The listing builds one solid part. Answer for the finished solid, in the listing's coordinates (mm). Face numbers are marked on the shaded views. A direction names the side the tool comes from. Coordinates: 2 decimals unless noted, no trailing zeros. Order: outer loops, then holes, each group sorted by start corner. A loop starts at its lowest first (then second) coordinate and runs counter-clockwise, first axis right, second up. Notation, with made-up numbers: (52.5, -15.75) -> (68.5, -15.75) arc R12 cw to (68.5, 0.25) -> close; hole circle Ø8 at (-35.75, 27). An arc over 180 degrees is marked (long way). Put each result on its own line as item: value. Start each with the question number.
Autodesk Inventor part; units mm, degrees
ref_plane "YZ Plane" through (0, 0, 0) normal (1, 0, 0) x (0, 1, 0)
ref_plane "XZ Plane" through (0, 0, 0) normal (0, 1, 0) x (-1, 0, 0)
ref_plane "XY Plane" through (0, 0, 0) normal (0, 0, 1) x (1, 0, 0)
sketch "Эскиз1" plane through (0, 0, 0) normal (0, 0, 1) x (1, 0, 0)
  line L0 (-26, 14.5) -> (26, 14.5)
  line L1 (26, 14.5) -> (26, -14.5)
  line L2 (26, -14.5) -> (-26, -14.5)
  line L3 (-26, -14.5) -> (-26, 14.5)
  line L4 (0, -20.3) -> (0, 20.3)
  line L5 (-36.4, 0) -> (36.4, 0)
  point P0 (0, 0)
  dimension "d0" = 29
  dimension "d1" = 52
extrude "Выдавливание1" add sketch "Эскиз1" along normal blind 2
sketch "Эскиз2" plane through (0, 0, 2) normal (0, 0, 1) x (1, 0, 0)
  line L0 (-26, 14.5) -> (-26, -14.5)
  line L1 (26, 14.5) -> (-26, 14.5)
  line L2 (26, -14.5) -> (26, 14.5)
  line L3 (-26, -14.5) -> (26, -14.5)
  line L4 (-26, 14.5) -> (26, 14.5)
  line L5 (26, 14.5) -> (26, -14.5)
  line L6 (26, -14.5) -> (-26, -14.5)
  line L7 (-26, -14.5) -> (-26, 14.5)
  line L8 (-25, 13.5) -> (25, 13.5)
  line L9 (25, 13.5) -> (25, -13.5)
  line L10 (25, -13.5) -> (-25, -13.5)
  line L11 (-25, -13.5) -> (-25, 13.5)
  point P0 (0, 0)
  dimension "d4" = 1
  dimension "d5" = 1
  dimension "d6" = 1
  dimension "d7" = 1
extrude "Выдавливание2" add sketch "Эскиз2" along normal blind 15
sketch "Эскиз3" plane through (0, 0, 17) normal (0, 0, 1) x (1, 0, 0)
  line L0 (-26, 14.5) -> (-26, -14.5)
  line L1 (-26, 14.5) -> (-26, 14.5)
  line L2 (-26, 14.5) -> (-26, -14.5)
  line L3 (-26, -14.5) -> (-26, -14.5)
  line L4 (-28, -12.5) -> (-28, 12.5)
  line L5 (26, 14.5) -> (-26, 14.5)
  line L6 (26, 14.5) -> (26, 14.5)
  line L7 (28, 12.5) -> (28, -12.5)
  line L8 (26, -14.5) -> (26, -14.5)
  line L9 (26, -14.5) -> (26, 14.5)
  arc A0 (-26, 14.5) -> (-28, 12.5) centre (-26, 12.5) ccw
  arc A1 (-28, -12.5) -> (-26, -14.5) centre (-26, -12.5) ccw
  arc A2 (26, -14.5) -> (28, -12.5) centre (26, -12.5) ccw
  arc A3 (28, 12.5) -> (26, 14.5) centre (26, 12.5) ccw
  line L10 (-26, 14.5) -> (26, 14.5)
  line L11 (26, -14.5) -> (26, 14.5)
  line L12 (-26, -14.5) -> (26, -14.5)
  line L13 (-26, -12.5) -> (-27, -12.5)
  line L14 (-27, -12.5) -> (-27, 12.5)
  line L15 (-27, 12.5) -> (-26, 12.5)
  line L16 (-26, 12.5) -> (-26, -12.5)
  line L17 (26, 12.5) -> (27, 12.5)
  line L18 (27, 12.5) -> (27, -12.5)
  line L19 (27, -12.5) -> (26, -12.5)
  line L20 (26, -12.5) -> (26, 12.5)
  line L21 (-25, 13.5) -> (25, 13.5)
  line L22 (-25, -13.5) -> (-25, 13.5)
  line L23 (-25, 13.5) -> (-25, -13.5)
  line L24 (-25, -13.5) -> (25, -13.5)
  line L25 (25, -13.5) -> (25, 13.5)
  line L26 (25, 13.5) -> (-25, 13.5)
  point P0 (0, 0)
  point P1 (25, 13.5)
  dimension "d10" = 2
  dimension "d11" = 2
  dimension "d12" = 2
  dimension "d13" = 2
  dimension "d14" = 1
  dimension "d15" = 1
extrude "Выдавливание3" add sketch "Эскиз3" along normal blind 2 contours L5 L9 L12 L0 | L0 L15 L14 L13 A1 L4 A0 | A3 L7 A2 L9 L19 L18 L17
properties part number "бокс стандартный"
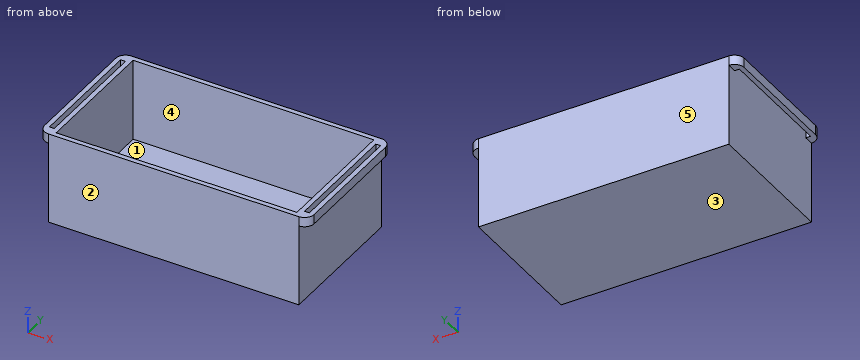
(1) The part is cut by section A-A on y = 3.25. Determine the outline of the cut face in (x, z), plus the area to 3 significant figures.
(2) A tool of negligible diameter and unlimited length cuts with its end or side. For the marked faces 4 and 5, from which of +Z, -Z, +X, -X, +Y, -Y can it reach the whole face along a straight path? Write none if from no direction.
(3) Find the intervals of material crossed by L1, parallel to X at y = 6, z = 7.5; L2, parallel to Y at x = -3, z = 6; L3, parallel to Z at x = 11.5, y = 6.5, in increasing order.
(4) Each of these flat-tipped pins is pushed along its axis until it touches: P1, Ø4, axis at y = -8.5, z = 3, coming from the -X side; P2, Ø4, axis at x = -19.5, y = -7, coming from the +Z side; P3, Ø0.8, axis at x = 26.5, z = 17.5, coming from the -Y side. Where does it stop, or does it pass through?
(5) For a pull along Y with two mould halves and no side action, classify the marked faces 1, 2 and 3 as released by +Y, released by -Y, zero draft, split by the parting line, or undercut.
(6) The part is cut by section B-B on z = 8.75. Determine the outline of the cut face in (x, y).
(7) The part is cut by section C-C on x = 19.5. Determine the outline of the cut face in (y, z).
Worked out:
1. outline: (-28, 17) -> (-27, 17) -> (-27, 19) -> (-28, 19) -> close; (-26, 0) -> (26, 0) -> (26, 19) -> (25, 19) -> (25, 2) -> (-25, 2) -> (-25, 19) -> (-26, 19) -> close; (27, 17) -> (28, 17) -> (28, 19) -> (27, 19) -> close
1. area: 142 mm2
2. face 4: +Z
2. face 5: +Z, -Z, +X, -X, +Y
3. L1: -26 to -25, 25 to 26
3. L2: -14.5 to -13.5, 13.5 to 14.5
3. L3: 0 to 2
4. P1: x = -26
4. P2: z = 2
4. P3: y = -14.5
5. face 1: undercut
5. face 2: released by -Y
5. face 3: zero draft
6. outline: (-26, -14.5) -> (26, -14.5) -> (26, 14.5) -> (-26, 14.5) -> close; hole (-25, -13.5) -> (25, -13.5) -> (25, 13.5) -> (-25, 13.5) -> close
7. outline: (-14.5, 0) -> (14.5, 0) -> (14.5, 19) -> (13.5, 19) -> (13.5, 2) -> (-13.5, 2) -> (-13.5, 19) -> (-14.5, 19) -> close
